from build123d import *

# Parameters (mm, degrees)
SKETCH1_W                       = 33
SKETCH1_H                       = 12
BOSS_EXTRUDE1_DEPTH             = 10
CBORE_FOR_M3_SBHCS1_D           = 3.6
CBORE_FOR_M3_SBHCS1_CBORE_D     = 6.7
CBORE_FOR_M3_SBHCS1_CBORE_DEPTH = 1.65


with BuildPart() as part:
    # Sketch1 → Boss-Extrude1 (new body)
    with BuildSketch(Plane(origin=(0, 0, 0), x_dir=(1, 0, 0), z_dir=(0, 1, 0))):
        Rectangle(SKETCH1_W, SKETCH1_H)
    extrude(amount=BOSS_EXTRUDE1_DEPTH)

    # Sketch1_4 one side → Cut-Revolve1 (revolve, cut)
    with BuildSketch(Plane(origin=(0, 0, 0), x_dir=(1, 0, 0), z_dir=(0, 1, 0))):
        Polygon((8, 3), (8, 6), (0, 6), (0, -6), (8, -6), (8, -3), (6, -3), (6, 3), align=None)
    revolve(axis=Axis((0, 0, -6), (0, 0, 1)), mode=Mode.SUBTRACT)

    # CBORE for M3 SBHCS1 (through all)
    with Locations(Plane(origin=(-12, 10, 0), x_dir=(0, 0, 1), z_dir=(0, 1, 0))):
        with Locations((0, 0), (0, 24)):
            CounterBoreHole(CBORE_FOR_M3_SBHCS1_D / 2, CBORE_FOR_M3_SBHCS1_CBORE_D / 2, CBORE_FOR_M3_SBHCS1_CBORE_DEPTH)


solid = part.part
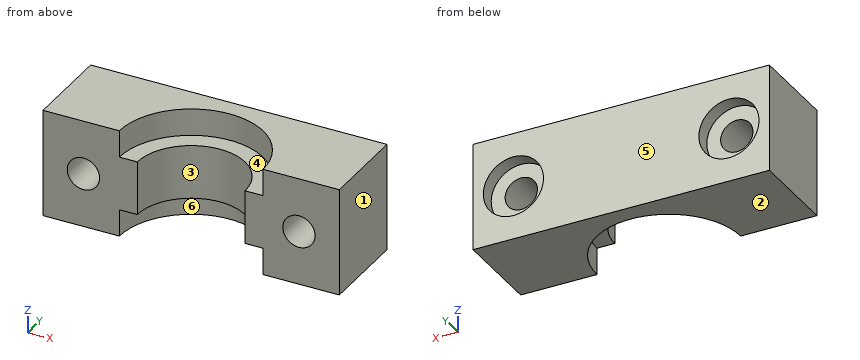
Model file for the job. Use its own axes, mm. Face numbers are marked on the shaded views. A direction names the side the tool comes from. Give positions to 0.01 mm unless a question says otherwise; leave off trailing zeros. Write each loop counter-clockwise with the first axis right and the second up, starting at its lowest first coordinate (ties: lowest second). Pieces come first, ordered by that corner, then holes. Notation, with made-up numbers: M 84.25,33 L 90.25,33 A22 cw 90.25,61 Z; hole C 8.25,-31 d4. An arc over 180 degrees is marked long. One line per item, written item: value. Start each with the question number.
Q1. Saw through at C-C, the plane x = -12. Write the cut outline in (y, z), plus the area to 3 significant figures.
Q2. Two-plate mould, pull along X, no slides. Class the marked faces 1, 2 and 3: +X half, -X half, draft (parallel to the pull), parting line (faces both ways), or undercut.
Q3. 3-axis set-ups, long thin cutter, end or side, ignore diameter. For the marked faces 4, 5 and 6: which of +Z, -Z, +X, -X, +Y, -Y reach the whole face in a straight line?
Q4. Drop flat-ended pins along their axis: pin 1 Ø4 at (x, y) = (-1, 3.5) entering from +Z; pin 2 Ø3.5 at (x, z) = (-12, 0.5) entering from +Y; pin 3 Ø1 at (x, y) = (-5.5, 2) entering from -Z. Give the stop position or say it passes through.
Q5. Saw through at B-B, the plane z = 0. Write the cut outline in (x, y), plus the area to 3 significant figures.
Q6. Probe probe 1 along X at (y, z) = (9.45, 0); probe 2 along Y at (x, z) = (-10.5, 2); probe 3 along X at (y, z) = (4.75, -3.25). List the from-to ranges inside material, lowest first. Write a range as [from, to].
Q7. Saw through at A-A, the plane y = 2.75. Write the cut outline in (x, z).
Q8. Saw through at D-D, the plane y = 9.5. Write the cut outline in (x, z), plus the area to 3 significant figures.
Output values:
1. outline: M 0,-6 L 10,-6 L 10,-3.35 L 8.35,-3.35 L 8.35,-1.8 L 0,-1.8 Z; M 0,1.8 L 8.35,1.8 L 8.35,3.35 L 10,3.35 L 10,6 L 0,6 Z
1. area: 78.9 mm²
2. face 1: +X half
2. face 2: draft
2. face 3: undercut
3. face 4: +Z, -Y
3. face 5: +Z, -Z, +X, -X, +Y
3. face 6: -Z, -Y
4. pin 1: passes through
4. pin 2: stops at y = 8.35
4. pin 3: stops at z = -3
5. outline: M -16.5,0 L -13.8,0 L -13.8,8.35 L -15.35,8.35 L -15.35,10 L -16.5,10 Z; M -10.2,0 L -6,0 A6 cw 6,0 L 10.2,0 L 10.2,8.35 L 8.65,8.35 L 8.65,10 L -8.65,10 L -8.65,8.35 L -10.2,8.35 Z; M 13.8,0 L 16.5,0 L 16.5,10 L 15.35,10 L 15.35,8.35 L 13.8,8.35 Z
5. area: 191 mm²
6. probe 1: x = [-16.5, -15.35], [-8.65, 8.65], [15.35, 16.5]
6. probe 2: y = [0, 8.35]
6. probe 3: x = [-16.5, -6.44], [6.44, 16.5]
7. outline: M -16.5,-6 L -7.51,-6 L -7.51,-3 L -5.33,-3 L -5.33,3 L -7.51,3 L -7.51,6 L -16.5,6 Z; M 5.33,-3 L 7.51,-3 L 7.51,-6 L 16.5,-6 L 16.5,6 L 7.51,6 L 7.51,3 L 5.33,3 Z; hole C -12,0 d3.6; hole C 12,0 d3.6
8. outline: M -16.5,-6 L 16.5,-6 L 16.5,6 L -16.5,6 Z; hole C -12,0 d6.7; hole C 12,0 d6.7
8. area: 325 mm²
